Can you work these out from the model? Positions are in its coordinate system, mm. Face numbers are marked on the shaded views. A direction names the side the tool comes from. Round coordinates to 2 decimals unless told otherwise and drop trailing zeros. Loops run counter-clockwise (first coordinate to the right, second up) from the corner with the lowest first, then second, coordinate; pieces in that order, holes last. Notation, with made-up numbers: (-0.75, 32) - (29.25, 32) arc R8 ccw to (29.25, 44) - close; hole circle Ø11 at (44.5, 10). An arc over 180 degrees is marked (long way). Answer as CSV lines item,"result".
```python
from build123d import *

# Parameters (mm, degrees)
F1_DEPTH = 25.4


with BuildPart() as f1:
    # F0 (on Top) → F1 (new body)
    with BuildSketch(Plane.XY):
        with BuildLine():
            Line((9.525, 9.525), (9.525, 12.7))
            Line((9.525, 12.7), (-9.525, 12.7))
            ThreePointArc((-9.525, 12.7), (-10.454936, 10.454936), (-12.7, 9.525))
            Line((-12.7, 9.525), (-12.7, -9.525))
            Line((-12.7, -9.525), (-9.525, -9.525))
            Line((-9.525, -9.525), (-9.525, -12.7))
            Line((-9.525, -12.7), (9.525, -12.7))
            ThreePointArc((9.525, -12.7), (10.156475, -10.156475), (12.7, -9.525))
            Line((12.7, -9.525), (12.7, 9.525))
            Line((12.7, 9.525), (9.525, 9.525))
        make_face()
        Polygon((-3.666174, 6.35), (3.666174, 6.35), (7.332348, 0), (3.666174, -6.35), (-3.666174, -6.35), (-7.332348, 0), align=None, mode=Mode.SUBTRACT)
    extrude(amount=F1_DEPTH)


solid = f1.part
```
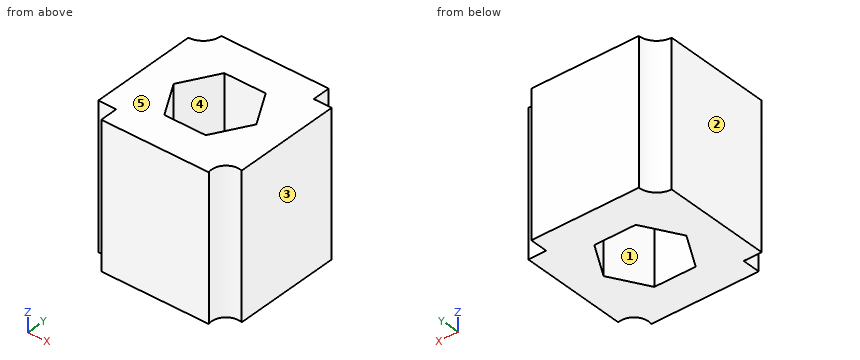
Q1. Imagine slicing it at B-B (y = -2.25). Write out the boundary of the cut face in (x, z).
Checks:
outline,"(-12.7, 0) - (-6.03, 0) - (-6.03, 25.4) - (-12.7, 25.4) - close; (6.03, 0) - (12.7, 0) - (12.7, 25.4) - (6.03, 25.4) - close"
Q2. We'd pull the mould along X, two halves only. Please class the marked faces 3, 4 and 5: pulls with the +X half, pulls with the -X half, needs draft (parallel to the pull), parting line crosses it, or undercut.
Checks:
face 3,"pulls with the +X half"
face 4,"undercut"
face 5,"needs draft"
Q3. Imagine slicing it at C-C (z = 9.25). Write out the boundary of the cut face in (x, y) (3 decimals).
Checks:
outline,"(-12.7, -9.525) - (-9.525, -9.525) - (-9.525, -12.7) - (9.525, -12.7) arc R2.54 cw to (12.7, -9.525) - (12.7, 9.525) - (9.525, 9.525) - (9.525, 12.7) - (-9.525, 12.7) arc R3.175 cw to (-12.7, 9.525) - close; hole (-7.332, 0) - (-3.666, -6.35) - (3.666, -6.35) - (7.332, 0) - (3.666, 6.35) - (-3.666, 6.35) - close"
Q4. If I drill on line 1 along Y through (x, z) = (3.25, 8.25); line 2 along Y through (x, z) = (5.5, 1.5); line 3 along X through (y, z) = (0, 7), over which ranges is the centre line in solid material (lowest first)? Write a range as [from, to].
Checks:
line 1,"[-12.7, -6.35], [6.35, 12.7]"
line 2,"[-12.7, -3.17], [3.17, 12.7]"
line 3,"[-12.7, -7.33], [7.33, 12.7]"
Q5. Imagine slicing it at A-A (x = -0.5). Write out the boundary of the cut face in (y, z).
Checks:
outline,"(-12.7, 0) - (-6.35, 0) - (-6.35, 25.4) - (-12.7, 25.4) - close; (6.35, 0) - (12.7, 0) - (12.7, 25.4) - (6.35, 25.4) - close"
Q6. I'm going to push flat-ended pins straight in: pin 1 Ø2.5 at (y, z) = (11, 16) entering from +X (3 decimals); pin 2 Ø1 at (y, z) = (-11, 9) entering from -X (3 decimals); pin 3 Ø1.6 at (x, z) = (10.5, 18) entering from +Y (3 decimals). Where does each tip first touch, or does it pass through?
Checks:
pin 1,"x = 9.525"
pin 2,"x = -9.525"
pin 3,"y = 9.525"
Q7. On a 3-axis mill with a long thin cutter (end or side, diameter ignored), from which of +Z, -Z, +X, -X, +Y, -Y can I reach the whole of each face in a straight line? I mean the marked faces 1 and 2. Say none if no direction works.
Checks:
face 1,"+Z, -Z"
face 2,"+Z, -Z, -X, +Y, -Y"
